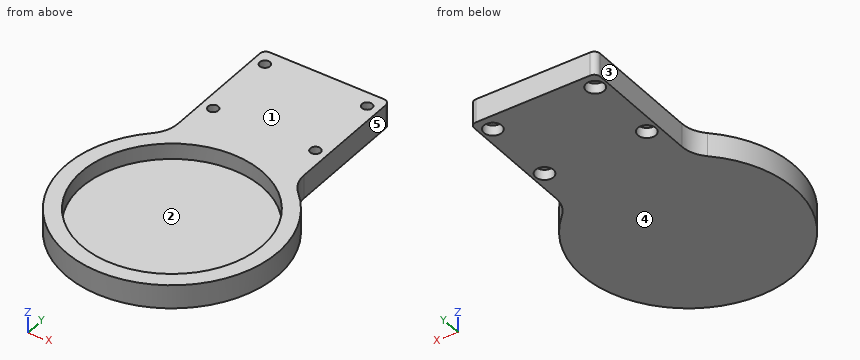
```python
from build123d import *

# Parameters (mm, degrees)
F0_R     = 36.5125
F1_DEPTH = 9.525
F2_R     = 36.5125
F3_DEPTH = 3.175
F4_R     = 2.0828
F5_DEPTH = 9.526
F6_R     = 3.6322
F6_R_2   = 2.0828
F7_DEPTH = 4.1656
F8_R     = 2.38125
F9_R     = 12.7


with BuildPart() as f1:
    # F0 (on Top) → F1 (new body)
    with BuildSketch(Plane.XY):
        with BuildLine():
            Line((-25.4, 90.5002), (-25.4, 34.525844))
            ThreePointArc((-25.4, 34.525844), (0, -42.8625), (25.4, 34.525844))
            Line((25.4, 34.525844), (25.4, 90.5002))
            Line((25.4, 90.5002), (-25.4, 90.5002))
        make_face()
        Circle(F0_R, mode=Mode.SUBTRACT)
    extrude(amount=F1_DEPTH)

    # F2 (on Top) → F3 (join)
    with BuildSketch(Plane.XY):
        Circle(F2_R)
    extrude(amount=F3_DEPTH)

    # F4 (on face) → F5 (cut, through all)
    with BuildSketch(Plane.XY.offset(9.525)):
        with Locations((-20.6375, 84.1502)):
            Circle(F4_R)
        with Locations((20.6375, 84.1502)):
            Circle(F4_R)
        with Locations((-20.6375, 53.975)):
            Circle(F4_R)
        with Locations((20.6375, 53.975)):
            Circle(F4_R)
    extrude(amount=-F5_DEPTH, mode=Mode.SUBTRACT)

    # F6 (on face) → F7 (cut)
    with BuildSketch(Plane.XY):
        with Locations((20.6375, 84.1502)):
            Circle(F6_R)
        with Locations((20.6375, 84.1502)):
            Circle(F6_R_2, mode=Mode.SUBTRACT)
        with Locations((-20.6375, 84.1502)):
            Circle(F6_R)
        with Locations((-20.6375, 84.1502)):
            Circle(F6_R_2, mode=Mode.SUBTRACT)
        with Locations((-20.6375, 53.975)):
            Circle(F6_R)
        with Locations((-20.6375, 53.975)):
            Circle(F6_R_2, mode=Mode.SUBTRACT)
        with Locations((20.6375, 53.975)):
            Circle(F6_R)
        with Locations((20.6375, 53.975)):
            Circle(F6_R_2, mode=Mode.SUBTRACT)
    extrude(amount=F7_DEPTH, mode=Mode.SUBTRACT)

    # F8
    f8_edges = [f1.edges().sort_by_distance(p)[0] for p in [
        (25.4, 90.5002, 4.7625),
        (-25.4, 90.5002, 4.7625),
    ]]
    fillet(f8_edges, radius=F8_R)

    # F9
    f9_edges = [f1.edges().sort_by_distance(p)[0] for p in [
        (25.4, 34.525844, 4.7625),
        (-25.4, 34.525844, 4.7625),
    ]]
    fillet(f9_edges, radius=F9_R)


solid = f1.part
```
Part model, mm, in its own coordinate system. Face numbers are marked on the shaded views. A direction names the side the tool comes from. Round coordinates to 2 decimals unless told otherwise and drop trailing zeros. Order: outer loops, then holes, each group sorted by start corner. A loop starts at its lowest first (then second) coordinate and runs counter-clockwise, first axis right, second up. Notation, with made-up numbers: M 69.5,22.25 L 74.5,22.25 A17 cw 74.5,53.25 Z; hole C 62.25,-16 d4. An arc over 180 degrees is marked long. Answer in a Markdown table with one row per item. Add a question column.
Q1. Cut at B-B on y = 0. Give the cut face in (x, z) (1 decimal).
Q2. Cut at A-A on x = 0. Give the cut face in (y, z) (1 decimal).
Q3. Pin check, flat tips, straight feed: pin 1 (1.5 mm diameter, centred on x = 20.5, z = 2.5, fed in from -Y); pin 2 (11.5 mm diameter, centred on x = -20.64, y = 53.98, fed in from +Z) (3 decimals); pin 3 (5 mm diameter, centred on x = 20.64, y = 84.15, fed in from -Z); pin 4 (8 mm diameter, centred on x = -6, y = 22.5, fed in from +Z) (3 decimals). Stop position of each tip, or through.
Q4. Mould opens along X. For the marked faces 1, 2 and 3 say: +X half, -X half, draft (parallel to the pull), parting line (faces both ways), or undercut.
Q5. Cut at D-D on x = 20. Give the cut face in (y, z) (3 decimals), and give its area (3 significant figures).
Q6. Wall check: L1, parallel to X at y = 83, z = 4; L2, parallel to X at y = 55, z = 5.25; L3, parallel to X at y = -1, z = 4.25. Give the ranges that are in metal, low to high. Write a range as from..to.
Q7. Cut at C-C on z = 7.75. Give the cut face in (x, y) (1 decimal), and give its area (3 significant figures).
Q8. 3-axis set-ups, long thin cutter, end or side, ignore diameter. For the marked faces 4 and 5: which of +Z, -Z, +X, -X, +Y, -Y reach the whole face in a straight line?
Established:
| question | item | result |
|---|---|---|
| 1 | outline | M -42.9,0 L 42.9,0 L 42.9,9.5 L 36.5,9.5 L 36.5,3.2 L -36.5,3.2 L -36.5,9.5 L -42.9,9.5 Z |
| 2 | outline | M -42.9,0 L 90.5,0 L 90.5,9.5 L 36.5,9.5 L 36.5,3.2 L -36.5,3.2 L -36.5,9.5 L -42.9,9.5 Z |
| 3 | pin 1 | stops at y = -38.04 |
| 3 | pin 2 | stops at z = 9.525 |
| 3 | pin 3 | stops at z = 4.17 |
| 3 | pin 4 | stops at z = 3.175 |
| 4 | face 1 | draft |
| 4 | face 2 | undercut |
| 4 | face 3 | -X half |
| 5 | outline | M -37.91,0 L 50.399,0 L 50.399,4.166 L 51.992,4.166 L 51.992,9.525 L 30.548,9.525 L 30.548,3.175 L -30.548,3.175 L -30.548,9.525 L -37.91,9.525 Z; M 55.958,4.166 L 57.551,4.166 L 57.551,0 L 80.574,0 L 80.574,4.166 L 82.167,4.166 L 82.167,9.525 L 55.958,9.525 Z; M 86.133,4.166 L 87.726,4.166 L 87.726,0 L 90.5,0 L 90.5,9.525 L 86.133,9.525 Z |
| 5 | area | 733 mm2 |
| 6 | L1 | x = -25.4..-24.08, -17.19..17.19, 24.08..25.4 |
| 6 | L2 | x = -25.4..-22.45, -18.82..18.82, 22.45..25.4 |
| 6 | L3 | x = -42.85..-36.5, 36.5..42.85 |
| 7 | outline | M -29.4,31.2 A42.9 ccw long 29.4,31.2 A12.7 cw 25.4,40.4 L 25.4,88.1 A2.4 ccw 23,90.5 L -23,90.5 A2.4 ccw -25.4,88.1 L -25.4,40.4 A12.7 cw Z; hole C 0,0 d73; hole C -20.6,54 d4.2; hole C -20.6,84.2 d4.2; hole C 20.6,54 d4.2; hole C 20.6,84.2 d4.2 |
| 7 | area | 4,090 mm2 |
| 8 | face 4 | -Z, +X, -X, +Y, -Y |
| 8 | face 5 | +Z, -Z, +X, +Y |
